The model under review builds one solid part; all positions refer to its coordinate system, in mm. Round coordinates to 2 decimals unless told otherwise and drop trailing zeros. Order: outer loops, then holes, each group sorted by start corner. A loop starts at its lowest first (then second) coordinate and runs counter-clockwise, first axis right, second up. Notation, with made-up numbers: M -31,6.5 L 23,6.5 A29 ccw 23,32.5 Z; hole C 45,76 d1. An arc over 180 degrees is marked long. Answer as a JSON object with one key per item and string values. Group by question number.
1) Consider section B-B, the plane z = 2.25. Write out the cut boundary in (x, y), then the cut area to 3 significant figures.
2) Consider section A-A, the plane x = 9.75. Write out the cut boundary in (y, z), then the cut area to 3 significant figures.
3) To check wall thickness, follow line 1 (X direction, y = -0.95, z = 9.75); line 2 (Z direction, x = -1.5, y = -3). State the ranges of each line that lie inside material, in increasing order.
4) Insertion check: pin 1 Ø0.7 at (y, z) = (-2.5, 2.5) entering from -X; pin 2 Ø1.5 at (x, y) = (1.5, -2) entering from +Z; pin 3 Ø1.2 at (y, z) = (-2, -3.5) entering from +X. Each pin has a flat end and moves straight along its axis. Give the tip position at first contact, or say it passes through.
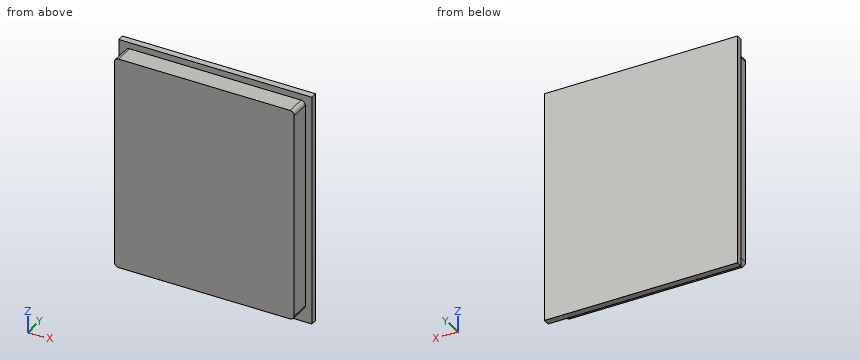
```python
from build123d import *

# Parameters (mm, degrees)
F0_W     = 23.3
F0_H     = 28
F1_DEPTH = 0.8
F2_W     = 21.7
F2_H     = 25.75
F3_DEPTH = 2.35
F4_R     = 0.5


with BuildPart() as f1:
    # F0 (on Front) → F1 (new body)
    with BuildSketch(Plane.XZ):
        Rectangle(F0_W, F0_H)
    extrude(amount=F1_DEPTH)

    # F2 (on face) → F3 (join)
    with BuildSketch(Plane.XZ.offset(0.8)):
        with Locations((0, 0.375)):
            Rectangle(F2_W, F2_H)
    extrude(amount=F3_DEPTH)

    # F4
    f4_edges = [f1.edges().sort_by_distance(p)[0] for p in [
        (-10.85, -1.975, -12.5),
        (10.85, -1.975, -12.5),
        (10.85, -1.975, 13.25),
        (-10.85, -1.975, 13.25),
    ]]
    fillet(f4_edges, radius=F4_R)


solid = f1.part
```
Results list:
{
 "1": {"outline": "M -11.65,-0.8 L -10.85,-0.8 L -10.85,-3.15 L 10.85,-3.15 L 10.85,-0.8 L 11.65,-0.8 L 11.65,0 L -11.65,0 Z", "area": "69.6 mm^2"},
 "2": {"outline": "M -3.15,-12.5 L -0.8,-12.5 L -0.8,-14 L 0,-14 L 0,14 L -0.8,14 L -0.8,13.25 L -3.15,13.25 Z", "area": "82.9 mm^2"},
 "3": {"line 1": "-10.85 to 10.85", "line 2": "-12.5 to 13.25"},
 "4": {"pin 1": "x = -10.85", "pin 2": "z = 13.25", "pin 3": "x = 10.85"}
}
